Input: part model. Units: mm. Frame: model coordinates. Face numbers are marked on the shaded views. Give positions to 0.01 mm unless a question says otherwise; leave off trailing zeros. Order: outer loops, then holes, each group sorted by start corner. A loop starts at its lowest first (then second) coordinate and runs counter-clockwise, first axis right, second up. Notation, with made-up numbers: (-15.75, 20.25) - (39.25, 20.25) arc R22 ccw to (39.25, 40.25) - close; hole circle Ø6 at (-10, 80.5). An arc over 180 degrees is marked (long way). Use a Markdown table: item, result.
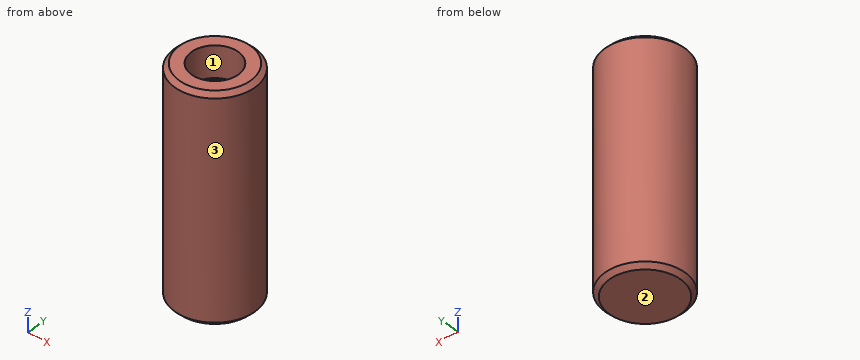
from build123d import *

# Parameters (mm, degrees)
F2_R     = 9
F3_DEPTH = 50
F4_R     = 5.25
F5_DEPTH = 7
F6_R     = 3.885
F7_DEPTH = 8.5
F10_SIZE = 1


with BuildPart() as f3:
    # F2 (on Top) → F3 (new body)
    with BuildSketch(Plane.XY):
        Circle(F2_R)
    extrude(amount=F3_DEPTH)

    # F4 (on face) → F5 (cut)
    with BuildSketch(Plane.XY.offset(50)):
        Circle(F4_R)
    extrude(amount=-F5_DEPTH, mode=Mode.SUBTRACT)

    # F6 (on face) → F7 (cut)
    with BuildSketch(Plane.XY.offset(43)):
        Circle(F6_R)
    extrude(amount=-F7_DEPTH, mode=Mode.SUBTRACT)

    # F8 (on Front) → F9 (revolve, cut)
    with BuildSketch(Plane.XZ):
        with BuildLine():
            ThreePointArc((0, 36.985), (-3.885, 33.1), (0, 29.215))
            Line((0, 29.215), (0, 36.985))
        make_face()
    revolve(axis=Axis((0, 0, 33.1), (0, 0, 1)), mode=Mode.SUBTRACT)

    # F10
    f10_edges = [f3.edges().sort_by_distance(p)[0] for p in [
        (-3.885, 0, 43),
        (-9, 0, 50),
        (-9, 0, 0),
    ]]
    chamfer(f10_edges, length=F10_SIZE)


solid = f3.part
1. Pin query (flat end, axial travel): pin 1 (8 mm diameter, centred on x = 6.5, z = 5, fed in from +Y); pin 2 (1 mm diameter, centred on y = 6, z = 10.5, fed in from +X); pin 3 (6 mm diameter, centred on x = 0, y = 0, fed in from +Z). Return the tip coordinate at first contact, or that it passes through.
Response:
| item | result |
|---|---|
| pin 1 | stops at y = 8.65 |
| pin 2 | stops at x = 7.12 |
| pin 3 | stops at z = 30.63 |
2. Section query D-D (z = 17). Return loops of the section in (x, y).
Response:
| item | result |
|---|---|
| outline | circle Ø18 at (0, 0) |
3. Material intervals for line 1 along Y through (x, z) = (0, 36.75) (3 decimals); line 2 along Y through (x, z) = (0, 46.5); line 3 along Y through (x, z) = (0, 16.5), sorted ascending.
Response:
| item | result |
|---|---|
| line 1 | y = -9 to -3.885, 3.885 to 9 |
| line 2 | y = -9 to -5.25, 5.25 to 9 |
| line 3 | y = -9 to 9 |
4. Section query B-B (x = 0). Return loops of the section in (y, z) (3 decimals).
Response:
| item | result |
|---|---|
| outline | (-9, 1) - (-8, 0) - (8, 0) - (9, 1) - (9, 49) - (8, 50) - (5.25, 50) - (5.25, 43) - (4.885, 43) - (3.885, 42) - (3.885, 34.5) - (3.624, 34.5) arc R3.885 cw (long way) to (-3.624, 34.5) - (-3.885, 34.5) - (-3.885, 42) - (-4.885, 43) - (-5.25, 43) - (-5.25, 50) - (-8, 50) - (-9, 49) - close |
5. Section query A-A (z = 37). Return loops of the section in (x, y) (3 decimals), then the cut area to 3 significant figures.
Response:
| item | result |
|---|---|
| outline | circle Ø18 at (0, 0); hole circle Ø7.77 at (0, 0) |
| area | 207 mm^2 |
6. Mould query, pull axis Y, two halves, no side actions, for the marked faces 1, 2 and 3. Classes: pulls with the +Y half, pulls with the -Y half, needs draft (parallel to the pull), parting line crosses it, or undercut.
Response:
| item | result |
|---|---|
| face 1 | undercut |
| face 2 | needs draft |
| face 3 | parting line crosses it |
